from build123d import *

# Parameters (mm, degrees)
F0_R            = 21.875
F0_R_2          = 11.25
F0_R_3          = 9.7
F1_DEPTH        = 2.4
F2_DEPTH        = 25
F3_D            = 5.5
F3_COPIES_COUNT = 3


# Not quite as in the source:
# - a pattern or mirror of a feature is missing from the dataset's text; its kind, count and spacing are read off the source's solid


with BuildPart() as f1:
    # F0 (on Top) → F1 (new body)
    with BuildSketch(Plane.XY):
        Circle(F0_R)
        Circle(F0_R_2, mode=Mode.SUBTRACT)
        Circle(F0_R_2)
        Circle(F0_R_3, mode=Mode.SUBTRACT)
    extrude(amount=F1_DEPTH)

    # F0 (on Top) → F2 (join)
    with BuildSketch(Plane.XY):
        Circle(F0_R_2)
        Circle(F0_R_3, mode=Mode.SUBTRACT)
    extrude(amount=F2_DEPTH)

    # F3 (through all)
    with Locations(Plane(origin=(0, 0, 0), x_dir=(1, 0, 0), z_dir=(0, 0, -1))):
        with Locations((-17.625, 0)):
            f3 = Hole(F3_D / 2)

    # F3_copies: F3 ×3 about axis
    f3_copies_axis = Axis((0, 0, 0), (0, 0, 1))
    for i in range(1, F3_COPIES_COUNT):
        add(f3.rotate(f3_copies_axis, i * 360 / F3_COPIES_COUNT), mode=Mode.SUBTRACT)


solid = f1.part
The listing builds one solid part. Answer for the finished solid, in the listing's coordinates (mm). A direction names the side the tool comes from. Give positions to 0.01 mm unless a question says otherwise; leave off trailing zeros. Write each loop counter-clockwise with the first axis right and the second up, starting at its lowest first coordinate (ties: lowest second). Pieces come first, ordered by that corner, then holes.
1) For a pull along Y with two mould halves and no side action, classify faces 3 (the face through (7.334, 12.945, 1.217)), 4 (the face through (9, -9, 2.4)), 5 (the face through (-16.123, 14.784, 1.183)), 6 (the face through (9.252, 2.914, 12.325)) as pulls with the +Y half, pulls with the -Y half, needs draft (parallel to the pull), parting line crosses it, or undercut.
2) Section B-B (y = 0) is taken. Write down the section's boundary in (x, z) (3 decimals), and give its area (3 significant figures).
3) Section D-D (x = 8) is taken. Write down the section's boundary in (y, z), and give its area (3 significant figures).
4) A tool of negligible diameter and unlimited length cuts with its end or side. For faces 1 (the face through (-14.878, -0.121, 1.217)), 2 (the face through (5.19, -9.98, 13.54)), from which of +Z, -Z, +X, -X, +Y, -Y can it reach the whole face along a straight path? Write none if from no direction.
5) Find the intervals of material crossed by L1, parallel to Y at x = 0, z = 11.75; L2, parallel to Z at x = -4, y = 19; L3, parallel to X at y = -6, z = 7.75, in increasing order.
6) Given P1, Ø2, axis at x = 10.5, y = 10, coming from the -Z side; P2, Ø1.5, axis at x = -9, z = 17, coming from the +Y side; P3, Ø3, axis at x = 3.5, z = 19, coming from the +Y side; P4, Ø8, axis at y = 1.5, z = 20, coming from the +X side, each flat-ended and moving along its own axis, determine where each tip first touches the part or whether it passes through.
7) Section A-A (x = 0) is taken. Write down the section's boundary in (y, z) (3 decimals).
8) Section C-C (y = 5.5) is taken. Write down the section's boundary in (x, z), and give its area (3 significant figures).
Response:
1. face 3: undercut
1. face 4: needs draft
1. face 5: parting line crosses it
1. face 6: undercut
2. outline: (-21.875, 0) - (-20.375, 0) - (-20.375, 2.4) - (-21.875, 2.4) - close; (-14.875, 0) - (-9.7, 0) - (-9.7, 25) - (-11.25, 25) - (-11.25, 2.4) - (-14.875, 2.4) - close; (9.7, 0) - (21.875, 0) - (21.875, 2.4) - (11.25, 2.4) - (11.25, 25) - (9.7, 25) - close
2. area: 115 mm2
3. outline: (-20.36, 0) - (-17.89, 0) - (-17.89, 2.4) - (-20.36, 2.4) - close; (-12.64, 0) - (-5.49, 0) - (-5.49, 25) - (-7.91, 25) - (-7.91, 2.4) - (-12.64, 2.4) - close; (5.49, 0) - (12.64, 0) - (12.64, 2.4) - (7.91, 2.4) - (7.91, 25) - (5.49, 25) - close; (17.89, 0) - (20.36, 0) - (20.36, 2.4) - (17.89, 2.4) - close
3. area: 156 mm2
4. face 1: +Z, -Z
4. face 2: +Z
5. L1: y = -11.25 to -9.7, 9.7 to 11.25
5. L2: z = 0 to 2.4
5. L3: x = -9.52 to -7.62, 7.62 to 9.52
6. P1: stops at z = 0
6. P2: stops at y = 7.65
6. P3: stops at y = 11.07
6. P4: stops at x = 11.25
7. outline: (-21.875, 0) - (-9.7, 0) - (-9.7, 25) - (-11.25, 25) - (-11.25, 2.4) - (-21.875, 2.4) - close; (9.7, 0) - (21.875, 0) - (21.875, 2.4) - (11.25, 2.4) - (11.25, 25) - (9.7, 25) - close
8. outline: (-21.17, 0) - (-7.99, 0) - (-7.99, 25) - (-9.81, 25) - (-9.81, 2.4) - (-21.17, 2.4) - close; (7.99, 0) - (21.17, 0) - (21.17, 2.4) - (9.81, 2.4) - (9.81, 25) - (7.99, 25) - close
8. area: 146 mm2
